Design review of the part built by this model. Coordinates are the model's own, in mm. A direction names the side the tool comes from. Coordinates: 2 decimals unless noted, no trailing zeros. Write each loop counter-clockwise with the first axis right and the second up, starting at its lowest first coordinate (ties: lowest second). Pieces come first, ordered by that corner, then holes. Notation, with made-up numbers: (81.5, 13.25) - (140.5, 13.25) arc R28 cw to (140.5, 40.25) - close; hole circle Ø4 at (19.25, 36.5). An arc over 180 degrees is marked (long way). Use a Markdown table: item, result.
from build123d import *

# Parameters (mm, degrees)
ESQUISSE1_R                = 3.6
ESQUISSE1_R_2              = 2.4
CC_AXE_SERVO_DEPTH         = 3.9
ESQUISSE3_R                = 2.7
ESQUISSE3_R_2              = 1.5
CC_PIVOT_JAMBE_DEPTH       = 3.9
ESQUISSE4_R                = 2.4
ESQUISSE4_R_2              = 1.5
LIAISON_DEPTH              = 4
ESQUISSE9_W                = 7
ESQUISSE9_H                = 1
ELASTICITE_AXE_SERVO_DEPTH = 5
ESQUISSE7_R                = 1.7
PASSAGE_VIS_DEPTH          = 5
ESQUISSE8_R                = 2.5
ESQUISSE8_R_2              = 1.7
BUTEE_ASSEMBLAGE_DEPTH     = 4
ESQUISSE10_W               = 5.2
ESQUISSE10_H               = 1
ELASTICITE_DEPTH           = 9


with BuildPart() as part:
    # Esquisse1 → CC_AXE_SERVO (new body)
    with BuildSketch(Plane.XY):
        Circle(ESQUISSE1_R)
        Circle(ESQUISSE1_R_2, mode=Mode.SUBTRACT)
    extrude(amount=CC_AXE_SERVO_DEPTH)



with BuildPart() as body_2:
    # Esquisse3 → CC_PIVOT_JAMBE (new body)
    with BuildSketch(Plane.XY):
        with Locations((40, 0)):
            Circle(ESQUISSE3_R)
        with Locations((40, 0)):
            Circle(ESQUISSE3_R_2, mode=Mode.SUBTRACT)
    extrude(amount=CC_PIVOT_JAMBE_DEPTH)


with BuildPart() as part_1:
    add(part.part)

    add(body_2.part)  # LIAISON merges body 2
    # Esquisse4 → LIAISON (add)
    with BuildSketch(Plane.XY):
        with BuildLine():
            Line((2.38117618, 2.7), (40, 2.7))
            ThreePointArc((40, 2.7), (42.7, 0), (40, -2.7))
            Line((40, -2.7), (2.38117618, -2.7))
            ThreePointArc((2.38117618, -2.7), (-3.6, 0), (2.38117618, 2.7))
        make_face()
        Circle(ESQUISSE4_R, mode=Mode.SUBTRACT)
        with Locations((40, 0)):
            Circle(ESQUISSE4_R_2, mode=Mode.SUBTRACT)
    extrude(amount=LIAISON_DEPTH)

    # Esquisse9 → ELASTICITE_AXE_SERVO (cut, through all)
    with BuildSketch(Plane.XY):
        with Locations((-0.1, 0)):
            Rectangle(ESQUISSE9_W, ESQUISSE9_H)
    extrude(amount=ELASTICITE_AXE_SERVO_DEPTH, mode=Mode.SUBTRACT)

    # Esquisse7 → PASSAGE_VIS (cut, through all)
    with BuildSketch(Plane.XY):
        with Locations((20, 0)):
            Circle(ESQUISSE7_R)
    extrude(amount=PASSAGE_VIS_DEPTH, mode=Mode.SUBTRACT)

    # Esquisse8 → BUTEE_ASSEMBLAGE (add)
    with BuildSketch(Plane.XY.offset(4)):
        with Locations((20, 0)):
            Circle(ESQUISSE8_R)
        with Locations((20, 0)):
            Circle(ESQUISSE8_R_2, mode=Mode.SUBTRACT)
    extrude(amount=BUTEE_ASSEMBLAGE_DEPTH)

    # Esquisse10 → ELASTICITE (cut, through all)
    with BuildSketch(Plane.XY):
        with Locations((40.1, 0)):
            Rectangle(ESQUISSE10_W, ESQUISSE10_H)
    extrude(amount=ELASTICITE_DEPTH, mode=Mode.SUBTRACT)


solid = part_1.part
(1) For pin 1 (1.4 mm diameter, centred on x = 42, z = 1.5, fed in from +Y); pin 2 (1 mm diameter, centred on x = 42.5, z = 1, fed in from -Y); pin 3 (1.3 mm diameter, centred on x = -3, z = 1.5, fed in from -Y), all flat-tipped, find the tip position at first contact; note any pin that passes through.
Determined:
| item | result |
|---|---|
| pin 1 | y = 2.37 |
| pin 2 | y = -1.81 |
| pin 3 | y = -2.73 |
(2) For L1, parallel to Y at x = 20, z = 3; L2, parallel to Y at x = 20, z = 7; L3, parallel to Z at x = 4, y = 0.75, list the stretches that pass through material, from the lowest coordinate up. Write a range as from..to.
Determined:
| item | result |
|---|---|
| L1 | -2.7..-1.7, 1.7..2.7 |
| L2 | -2.5..-1.7, 1.7..2.5 |
| L3 | 0..4 |
(3) Take a section at A-A on y = 0. Write out the cut boundary in (x, z), and give its area (3 significant figures).
Determined:
| item | result |
|---|---|
| outline | (3.4, 0) - (18.3, 0) - (18.3, 8) - (17.5, 8) - (17.5, 4) - (3.4, 4) - close; (21.7, 0) - (37.5, 0) - (37.5, 4) - (22.5, 4) - (22.5, 8) - (21.7, 8) - close |
| area | 129 mm2 |
(4) Take a section at D-D on x = 6.5. Write out the cut boundary in (y, z), and give its area (3 significant figures).
Determined:
| item | result |
|---|---|
| outline | (-2.7, 0) - (2.7, 0) - (2.7, 4) - (-2.7, 4) - close |
| area | 21.6 mm2 |
(5) Take a section at C-C on x = 20. Write out the cut boundary in (y, z), and give its area (3 significant figures).
Determined:
| item | result |
|---|---|
| outline | (-2.7, 0) - (-1.7, 0) - (-1.7, 8) - (-2.5, 8) - (-2.5, 4) - (-2.7, 4) - close; (1.7, 0) - (2.7, 0) - (2.7, 4) - (2.5, 4) - (2.5, 8) - (1.7, 8) - close |
| area | 14.4 mm2 |
(6) Take a section at B-B on z = 1.5. Write out the cut boundary in (x, y).
Determined:
| item | result |
|---|---|
| outline | (-3.57, -0.5) arc R3.6 ccw to (2.38, -2.7) - (40, -2.7) arc R2.7 ccw to (42.65, -0.5) - (41.41, -0.5) arc R1.5 cw to (38.59, -0.5) - (37.5, -0.5) - (37.5, 0.5) - (38.59, 0.5) arc R1.5 cw to (41.41, 0.5) - (42.65, 0.5) arc R2.7 ccw to (40, 2.7) - (2.38, 2.7) arc R3.6 ccw to (-3.57, 0.5) - (-2.35, 0.5) arc R2.4 cw to (2.35, 0.5) - (3.4, 0.5) - (3.4, -0.5) - (2.35, -0.5) arc R2.4 cw to (-2.35, -0.5) - close; hole circle Ø3.4 at (20, 0) |
(7) Machinability: for faces 5 (the flat face through (42, 0.5, 2)), 6 (the cylindrical face through (40, 1.5, 2)), 7 (the flat face through (-3, -0.5, 2)), which of the approach directions +Z, -Z, +X, -X, +Y, -Y give a long, thin tool a straight path to every point of the face, cutting with its end or side? Answer none if there is none.
Determined:
| item | result |
|---|---|
| face 5 | +Z, -Z, +X |
| face 6 | +Z, -Z |
| face 7 | +Z, -Z, -X |
(8) Draft analysis for pull direction X (two halves, no side actions). For faces 1 (the flat face through (38, 0.5, 2)), 2 (the cylindrical face through (40, -1.5, 2)), 3 (the cylindrical face through (17.5, 0.1, 6)), 4 (the flat face through (3.4, 0, 2)), state which applies: +X half, -X half, draft (parallel to the pull), parting line (faces both ways), or undercut.
Determined:
| item | result |
|---|---|
| face 1 | draft |
| face 2 | undercut |
| face 3 | parting line |
| face 4 | -X half |
